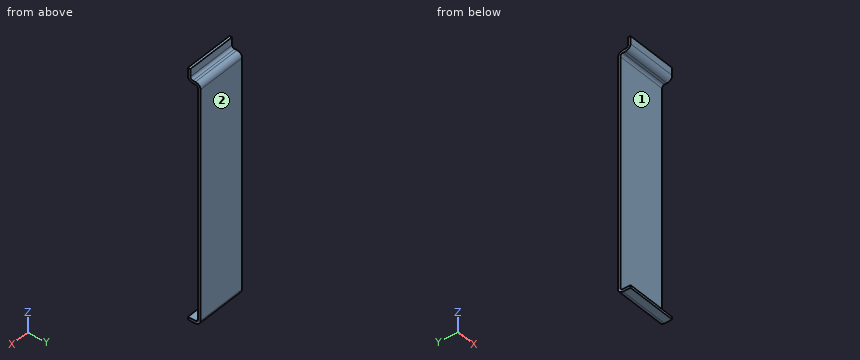
from build123d import *

# Parameters (mm, degrees)
ESBO_O1_W                      = 40
ESBO_O1_H                      = 180
FLANGE_BASE1_DEPTH             = 2
ARESTA_FLANGE1_DEPTH           = 40
ARESTA_FLANGE1_BEND_DEPTH      = 40
ARESTA_FLANGE4_STRIP_W         = 12
ARESTA_FLANGE4_STRIP_H         = 2
ARESTA_FLANGE4_STRIP_CUT_DEPTH = 40
ARESTA_FLANGE4_DEPTH           = 40


# Sheet-metal steps are written as plain solids
with BuildPart() as part:
    # Esboço1 → Flange-base1 (new body)
    with BuildSketch(Plane(origin=(0, 0, 0), x_dir=(1, 0, 0), z_dir=(0, 1, 0))):
        Rectangle(ESBO_O1_W, ESBO_O1_H)
    extrude(amount=-FLANGE_BASE1_DEPTH)

    # Aresta-Flange1 section (across the edge) → Aresta-Flange1 (add)
    with BuildSketch(Plane(origin=(20, -2, 92), x_dir=(0, 0, -1), z_dir=(-1, 0, 0))):
        with BuildLine():
            Line((-2, 2), (-2, 8))
            Line((-2, 8), (0, 8))
            Line((0, 8), (0, 2))
            ThreePointArc((0, 2), (0.585786438, 0.585786438), (2, 0))
            Line((2, 0), (2, -2))
            ThreePointArc((2, -2), (-0.828427125, -0.828427125), (-2, 2))
        make_face()
    extrude(amount=ARESTA_FLANGE1_DEPTH)

    # Aresta-Flange1 section 2 (across the edge) → Aresta-Flange1 bend (add)
    with BuildSketch(Plane(origin=(-20, -2, -92), x_dir=(0, 0, 1), z_dir=(1, 0, 0))):
        with BuildLine():
            Line((-2, 2), (-2, 8))
            Line((-2, 8), (0, 8))
            Line((0, 8), (0, 2))
            ThreePointArc((0, 2), (0.585786438, 0.585786438), (2, 0))
            Line((2, 0), (2, -2))
            ThreePointArc((2, -2), (-0.828427125, -0.828427125), (-2, 2))
        make_face()
    extrude(amount=ARESTA_FLANGE1_BEND_DEPTH)

    # Aresta-Flange4 strip (across the edge) → Aresta-Flange4 strip cut (cut)
    with BuildSketch(Plane(origin=(-20, -10, 94), x_dir=(0, 1, 0), z_dir=(1, 0, 0))):
        with Locations((-2, -1)):
            Rectangle(ARESTA_FLANGE4_STRIP_W, ARESTA_FLANGE4_STRIP_H)
    extrude(amount=ARESTA_FLANGE4_STRIP_CUT_DEPTH, mode=Mode.SUBTRACT)

    # Aresta-Flange4 section (across the edge) → Aresta-Flange4 (add)
    with BuildSketch(Plane(origin=(-20, -10, 94), x_dir=(0, 1, 0), z_dir=(1, 0, 0))):
        with BuildLine():
            Line((0, 2), (0, 8))
            Line((0, 8), (2, 8))
            Line((2, 8), (2, 2))
            ThreePointArc((2, 2), (2.585786438, 0.585786438), (4, 0))
            Line((4, 0), (4, -2))
            ThreePointArc((4, -2), (1.171572875, -0.828427125), (0, 2))
        make_face()
    extrude(amount=ARESTA_FLANGE4_DEPTH)


solid = part.part
Input: part model. Units: mm. Frame: model coordinates. Face numbers are marked on the shaded views. A direction names the side the tool comes from. Coordinates: 2 decimals unless noted, no trailing zeros. Order: outer loops, then holes, each group sorted by start corner. A loop starts at its lowest first (then second) coordinate and runs counter-clockwise, first axis right, second up. Notation, with made-up numbers: M 3.25,-38.5 L 43.25,-38.5 A21 cw 43.25,-21.5 Z; hole C -37,78.5 d5. An arc over 180 degrees is marked long. One line per question, with ' | ' between items.
Item 1: Section B-B (z = -48). Output: boundary loops of the cut face in (x, y), then the cut area to 3 significant figures.
Geometry results:
outline: M -20,-2 L 20,-2 L 20,0 L -20,0 Z | area: 80.0 mm^2
Item 2: Pin query (flat end, axial travel): pin 1 (1.5 mm diameter, centred on x = -3, y = -2, fed in from -Z); pin 2 (6.5 mm diameter, centred on x = -4.5, z = 98.5, fed in from +Y); pin 3 (6 mm diameter, centred on x = 3.5, y = -4.5, fed in from +Z). Return the tip coordinate at first contact, or that it passes through.
Geometry results:
pin 1: stops at z = -93.8 | pin 2: stops at y = -7.85 | pin 3: stops at z = 94.68
Item 3: Section A-A (x = -16.5). Output: boundary loops of the cut face in (y, z).
Geometry results:
outline: M -10,-94 L -4,-94 A4 ccw 0,-90 L 0,90 A4 ccw -4,94 L -6,94 A2 cw -8,96 L -8,102 L -10,102 L -10,96 A4 ccw -6,92 L -4,92 A2 cw -2,90 L -2,-90 A2 cw -4,-92 L -10,-92 Z
Item 4: Reachability of the marked faces 1 and 2 from +Z, -Z, +X, -X, +Y, -Y: full face, straight path, thin tool, end or side. Return the list, or none.
Geometry results:
face 1: +X, -X, -Y | face 2: +Z, -Z, +X, -X, +Y
Item 5: Ray query, line 1 along Z through (x, y) = (-8.5, -3.75); line 2 along Y through (x, z) = (-12.5, 66); line 3 along Z through (x, y) = (-12, -2.75). Return the intervals inside material, ascending.
Geometry results:
line 1: z = -93.99 to -91.98, 91.98 to 93.99 | line 2: y = -2 to 0 | line 3: z = -93.8 to -91.56, 91.56 to 93.8
